from build123d import *

# Parameters (mm, degrees)
SKETCH1_W           = 100
SKETCH1_H           = 100
BOSS_EXTRUDE1_DEPTH = 4
SKETCH2_R           = 4.7625
CUT_EXTRUDE1_DEPTH  = 71.823724839
SKETCH3_W           = 8.5
SKETCH3_H           = 8.5
CUT_EXTRUDE2_DEPTH  = 71.823724839
BOSS_EXTRUDE3_DEPTH = 29
BOSS_EXTRUDE4_DEPTH = 29
CUT_EXTRUDE4_DEPTH  = 77.426435217
BOSS_EXTRUDE5_DEPTH = 29
BOSS_EXTRUDE6_DEPTH = 29
SKETCH12_R          = 1.5
CUT_EXTRUDE5_DEPTH  = 79.0320447
CUT_EXTRUDE6_DEPTH  = 3
SKETCH15_R          = 1.5
CUT_EXTRUDE7_DEPTH  = 10


with BuildPart() as part:
    # Sketch1 → Boss-Extrude1 (new body)
    with BuildSketch(Plane(origin=(0, 0, 0), x_dir=(1, 0, 0), z_dir=(0, 1, 0))):
        Rectangle(SKETCH1_W, SKETCH1_H)
    extrude(amount=BOSS_EXTRUDE1_DEPTH)

    # Sketch2 → Cut-Extrude1 (cut, through all)
    with BuildSketch(Plane(origin=(0, 4, 0), x_dir=(1, 0, 0), z_dir=(0, 1, 0))):
        with Locations(Location((0, 0, 0), (0, 0, 270))):
            Circle(SKETCH2_R)
    extrude(amount=-CUT_EXTRUDE1_DEPTH, mode=Mode.SUBTRACT)

    # Sketch3 → Cut-Extrude2 (cut, through all)
    with BuildSketch(Plane(origin=(0, 4, 0), x_dir=(1, 0, 0), z_dir=(0, 1, 0))):
        with Locations((-45.75, 45.75)):
            Rectangle(SKETCH3_W, SKETCH3_H)
        with Locations((45.75, 45.75)):
            Rectangle(SKETCH3_W, SKETCH3_H)
        with Locations((45.75, -45.75)):
            Rectangle(SKETCH3_W, SKETCH3_H)
        with Locations((-45.75, -45.75)):
            Rectangle(SKETCH3_W, SKETCH3_H)
    extrude(amount=-CUT_EXTRUDE2_DEPTH, mode=Mode.SUBTRACT)

    # Sketch4 → Boss-Extrude3 (add)
    with BuildSketch(Plane(origin=(0, 4, 0), x_dir=(1, 0, 0), z_dir=(0, 1, 0))):
        with BuildLine():
            Line((-10.927389365, -13.022755533), (-11.891570779, -14.171822198))
            ThreePointArc((-11.891570779, -14.171822198), (0, -18.5), (11.891570779, -14.171822198))
            Line((11.891570779, -14.171822198), (10.927389365, -13.022755533))
            ThreePointArc((10.927389365, -13.022755533), (0, -17), (-10.927389365, -13.022755533))
        make_face()
        with BuildLine():
            Line((-13.022755533, -10.927389365), (-14.171822198, -11.891570779))
            ThreePointArc((-14.171822198, -11.891570779), (-18.5, 0), (-14.171822198, 11.891570779))
            Line((-14.171822198, 11.891570779), (-13.022755533, 10.927389365))
            ThreePointArc((-13.022755533, 10.927389365), (-17, 0), (-13.022755533, -10.927389365))
        make_face()
        with BuildLine():
            Line((-10.927389365, 13.022755533), (-11.891570779, 14.171822198))
            ThreePointArc((-11.891570779, 14.171822198), (0, 18.5), (11.891570779, 14.171822198))
            Line((11.891570779, 14.171822198), (10.927389365, 13.022755533))
            ThreePointArc((10.927389365, 13.022755533), (0, 17), (-10.927389365, 13.022755533))
        make_face()
        with BuildLine():
            Line((13.022755533, 10.927389365), (14.171822198, 11.891570779))
            ThreePointArc((14.171822198, 11.891570779), (18.5, 0), (14.171822198, -11.891570779))
            Line((14.171822198, -11.891570779), (13.022755533, -10.927389365))
            ThreePointArc((13.022755533, -10.927389365), (17, 0), (13.022755533, 10.927389365))
        make_face()
    extrude(amount=BOSS_EXTRUDE3_DEPTH)

    # Sketch7 → Boss-Extrude4 (add)
    with BuildSketch(Plane(origin=(0, 4, 0), x_dir=(1, 0, 0), z_dir=(0, 1, 0))):
        Polygon((-41.5, -41.5), (-41.5, -50), (-40, -50), (-40, -40), (-50, -40), (-50, -41.5), align=None)
        Polygon((40, -50), (40, -40), (50, -40), (50, -41.5), (41.5, -41.5), (41.5, -50), align=None)
        Polygon((50, 41.5), (50, 40), (40, 40), (40, 50), (41.5, 50), (41.5, 41.5), align=None)
        Polygon((-50, 41.5), (-50, 40), (-40, 40), (-40, 50), (-41.5, 50), (-41.5, 41.5), align=None)
    extrude(amount=BOSS_EXTRUDE4_DEPTH)

    # Sketch8 → Cut-Extrude4 (cut, through all)
    with BuildSketch(Plane(origin=(0, 4, 0), x_dir=(1, 0, 0), z_dir=(0, 1, 0))):
        Polygon((-14.171822198, -11.891570779), (-40, -50), (-36.17429682, -50), (-11.891570779, -14.171822198), (-9.867198001, -11.184942236), (-12.488706492, -9.408201793), align=None)
        Polygon((-11.891570779, 14.171822198), (-50, 40), (-50, 36.17429682), (-14.171822198, 11.891570779), (-11.184942236, 9.867198001), (-9.408201793, 12.488706492), align=None)
        Polygon((14.171822198, 11.891570779), (40, 50), (36.17429682, 50), (11.891570779, 14.171822198), (9.867198001, 11.184942236), (12.488706492, 9.408201793), align=None)
        Polygon((11.891570779, -14.171822198), (50, -40), (50, -36.17429682), (14.171822198, -11.891570779), (11.184942236, -9.867198001), (9.408201793, -12.488706492), align=None)
    extrude(amount=CUT_EXTRUDE4_DEPTH, mode=Mode.SUBTRACT)

    # Sketch9 → Boss-Extrude5 (add)
    with BuildSketch(Plane(origin=(0, 4, 0), x_dir=(1, 0, 0), z_dir=(0, 1, 0))):
        Polygon((-11.891570779, -14.171822198), (-36.17429682, -50), (-34.17429682, -50), (-10.52109933, -15.100666052), align=None)
        Polygon((-14.171822198, -11.891570779), (-40, -50), (-40, -47.049081084), (-14.981255079, -10.134937263), (-13.610783629, -11.063781117), align=None)
        Polygon((-50, 34.17429682), (-15.100666052, 10.52109933), (-14.171822198, 11.891570779), (-50, 36.17429682), align=None)
        Polygon((-11.891570779, 14.171822198), (-50, 40), (-47.049081084, 40), (-10.134937263, 14.981255079), (-11.063781117, 13.610783629), align=None)
        Polygon((34.17429682, 50), (10.52109933, 15.100666052), (11.891570779, 14.171822198), (36.17429682, 50), align=None)
        Polygon((14.171822198, 11.891570779), (40, 50), (40, 47.049081084), (14.981255079, 10.134937263), (13.610783629, 11.063781117), align=None)
        Polygon((50, -34.17429682), (15.100666052, -10.52109933), (14.171822198, -11.891570779), (50, -36.17429682), align=None)
        Polygon((11.891570779, -14.171822198), (50, -40), (47.049081084, -40), (10.134937263, -14.981255079), (11.063781117, -13.610783629), align=None)
    extrude(amount=BOSS_EXTRUDE5_DEPTH)

    # Sketch11 → Boss-Extrude6 (add)
    with BuildSketch(Plane(origin=(0, 4, 0), x_dir=(1, 0, 0), z_dir=(0, 1, 0))):
        Polygon((-40, -40), (-35.222450169, -40), (-40, -47.049081084), align=None)
        Polygon((-40, 40), (-40, 35.222450169), (-47.049081084, 40), align=None)
        Polygon((40, 40), (35.222450169, 40), (40, 47.049081084), align=None)
        Polygon((40, -40), (40, -35.222450169), (47.049081084, -40), align=None)
    extrude(amount=BOSS_EXTRUDE6_DEPTH)

    # Sketch12 → Cut-Extrude5 (cut, through all)
    with BuildSketch(Plane(origin=(0, 0, 0), x_dir=(-1, 0, 0), z_dir=(0, -1, 0))):
        with Locations(Location((-3.5, 33, 0), (0, 0, 90))):
            Circle(SKETCH12_R)
        with Locations(Location((-3.5, -33, 0), (0, 0, 90))):
            Circle(SKETCH12_R)
        with Locations(Location((-35, 33, 0), (0, 0, 90))):
            Circle(SKETCH12_R)
        with Locations(Location((-28, -33, 0), (0, 0, 90))):
            Circle(SKETCH12_R)
    extrude(amount=-CUT_EXTRUDE5_DEPTH, mode=Mode.SUBTRACT)

    # Sketch14 → Cut-Extrude6 (cut)
    with BuildSketch(Plane(origin=(0, 4, 0), x_dir=(1, 0, 0), z_dir=(0, 1, 0))):
        Polygon((28, -29.882308546), (25.3, -31.441154273), (25.3, -34.558845727), (28, -36.117691454), (30.7, -34.558845727), (30.7, -31.441154273), align=None)
        Polygon((3.5, -29.882308546), (0.8, -31.441154273), (0.8, -34.558845727), (3.5, -36.117691454), (6.2, -34.558845727), (6.2, -31.441154273), align=None)
        Polygon((3.5, 36.117691454), (0.8, 34.558845727), (0.8, 31.441154273), (3.5, 29.882308546), (6.2, 31.441154273), (6.2, 34.558845727), align=None)
        Polygon((35, 36.117691454), (32.3, 34.558845727), (32.3, 31.441154273), (35, 29.882308546), (37.7, 31.441154273), (37.7, 34.558845727), align=None)
    extrude(amount=-CUT_EXTRUDE6_DEPTH, mode=Mode.SUBTRACT)

    # Sketch15 → Cut-Extrude7 (cut)
    with BuildSketch(Plane(origin=(0, 33, 0), x_dir=(1, 0, 0), z_dir=(0, 1, 0))):
        with Locations(Location((44, -39, 0), (0, 0, 270))):
            Circle(SKETCH15_R)
        with Locations(Location((-39, -44, 0), (0, 0, 270))):
            Circle(SKETCH15_R)
        with Locations(Location((-44, 39, 0), (0, 0, 270))):
            Circle(SKETCH15_R)
        with Locations(Location((39, 44, 0), (0, 0, 270))):
            Circle(SKETCH15_R)
    extrude(amount=-CUT_EXTRUDE7_DEPTH, mode=Mode.SUBTRACT)


solid = part.part
Verification items for the finished model (mm, model axes). A direction names the side the tool comes from. Give positions to 0.01 mm unless a question says otherwise; leave off trailing zeros. Loops run counter-clockwise (first coordinate to the right, second up) from the corner with the lowest first, then second, coordinate; pieces in that order, holes last.
1) Draft check along X on faces 6 (the flat face through (23.863, 18.297, -31.835)), 7 (the cylindrical face through (-39.9, 28.1, 42.8)), 8 (the flat face through (-9, 3, 50)), 9 (the flat face through (-50, 3, -9)). Enter one of: pulls with the +X half, pulls with the -X half, needs draft (parallel to the pull), parting line crosses it, or undercut.
2) Sectioned sample at B-B, the plane x = 44. Enter the section's corners in (y, z).
3) Sectioned sample at A-A, the plane y = 10. Count the separate pieces of the cut face and the enclosed holes in it, then the cut area to 3 significant figures.
4) Set-up check for faces 1 (the flat face through (-41.5, 16, 46)), 2 (the flat face through (-43, 18, 40)), 3 (the flat face through (2.17, 2.52, -35.35)), 4 (the flat face through (2, 4, 36)), 5 (the flat face through (-3, 4, -37)): record each of +Z, -Z, +X, -X, +Y, -Y from which the full face is reachable in a straight line by a thin tool's end or side.
5) Thickness scan on line 1 along X through (y, z) = (0.65, 33); line 2 along X through (y, z) = (0.3, -33); line 3 along X through (y, z) = (23, -28.5). Record the ranges inside material, lowest first.
6) Sectioned sample at C-C, the plane z = 44. Enter the section's corners in (x, y), then the cut area to 3 significant figures.
7) Depth check by flat-ended pin: pin 1 Ø12 at (x, z) = (-30.5, 18.5) entering from -Y; pin 2 Ø12 at (y, z) = (29.5, -20.5) entering from -X; pin 3 Ø5 at (y, z) = (11.5, 23) entering from +X; pin 4 Ø4 at (x, y) = (47.5, 9) entering from -Z. Enter the tip coordinate at first touch or a pass-through.
Answers:
1. face 6: undercut
1. face 7: undercut
1. face 8: needs draft
1. face 9: pulls with the -X half
2. outline: (0, -41.5) - (33, -41.5) - (33, -40) - (4, -40) - (4, 30.11) - (33, 30.11) - (33, 32.11) - (4, 32.11) - (4, 35.93) - (33, 35.93) - (33, 37.5) - (23, 37.5) - (23, 40.5) - (33, 40.5) - (33, 41.5) - (0, 41.5) - close
3. separate pieces: 4
3. enclosed holes: 0
3. area: 907 mm2
4. face 1: +Z, -X, +Y, -Y
4. face 2: -X, +Y
4. face 3: +Y
4. face 4: +Z, +Y
4. face 5: -Z, +Y
5. line 1: x = -50 to 2, 5 to 26.5, 29.5 to 50
5. line 2: x = -50 to 2, 5 to 33.5, 36.5 to 50
5. line 3: x = -41.63 to -38.68, -33.03 to -30.08, 19.6 to 21.6, 25.43 to 27.43
6. outline: (-41.5, 0) - (41.5, 0) - (41.5, 33) - (40, 33) - (40, 4) - (-30.11, 4) - (-30.11, 33) - (-32.11, 33) - (-32.11, 4) - (-35.93, 4) - (-35.93, 33) - (-37.5, 33) - (-37.5, 23) - (-40.5, 23) - (-40.5, 33) - (-41.5, 33) - close
6. area: 565 mm2
7. pin 1: stops at y = 0
7. pin 2: stops at x = -38.68
7. pin 3: stops at x = 37.2
7. pin 4: stops at z = -41.5
